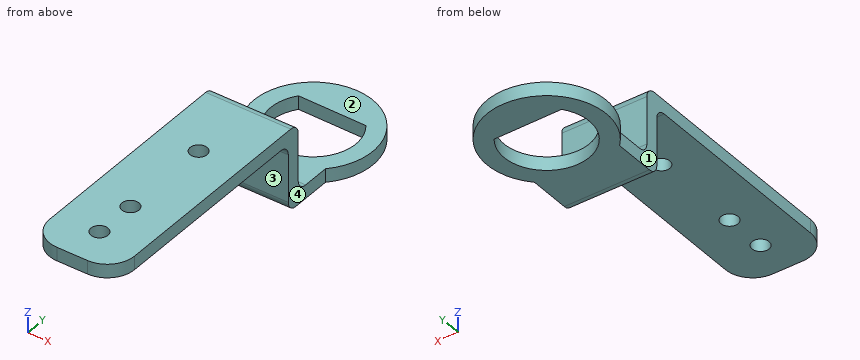
```python
from build123d import *

# Parameters (mm, degrees)
BOSS_EXTRUDE1_DEPTH = 0.4
SKETCH2_W           = 2.5
SKETCH2_H           = 0.4
BOSS_EXTRUDE2_DEPTH = 2
SKETCH3_W           = 2.5
SKETCH3_H           = 0.4
BOSS_EXTRUDE3_DEPTH = 7
FILLET1_R           = 0.3
FILLET2_R           = 0.8
SKETCH4_R           = 0.25
CUT_EXTRUDE1_DEPTH  = 4


with BuildPart() as part:
    # Sketch1 → Boss-Extrude1 (new body)
    with BuildSketch(Plane.XY):
        with BuildLine():
            Line((0.266025337, -2.019252852), (0.266025337, -3.519252852))
            Line((0.266025337, -3.519252852), (2.766025337, -3.519252852))
            Line((2.766025337, -3.519252852), (2.766025337, -2.019252852))
            ThreePointArc((2.766025337, -2.019252852), (1.516025337, 0.955492019), (0.266025337, -2.019252852))
        make_face()
        with BuildLine():
            Line((2.524676695, -0.056183906), (0.524811845, -0.032933419))
            ThreePointArc((0.524811845, -0.032933419), (1.501493783, -2.044423511), (2.524676695, -0.056183906))
        make_face(mode=Mode.SUBTRACT)
    extrude(amount=BOSS_EXTRUDE1_DEPTH)

    # Sketch2 → Boss-Extrude2 (add)
    with BuildSketch(Plane.XY.offset(0.4)):
        with Locations((1.516025337, -3.319252852)):
            Rectangle(SKETCH2_W, SKETCH2_H)
    extrude(amount=BOSS_EXTRUDE2_DEPTH)

    # Sketch3 → Boss-Extrude3 (add)
    with BuildSketch(Plane.XZ.offset(3.519252852)):
        with Locations((1.516025337, 2.2)):
            Rectangle(SKETCH3_W, SKETCH3_H)
    extrude(amount=BOSS_EXTRUDE3_DEPTH)

    # Fillet1
    fillet1_edges = [part.edges().sort_by_distance(p)[0] for p in [
        (1.516025337, -3.119252852, 0.4),
        (1.516025337, -3.119252852, 2.4),
        (1.516025337, -3.519252852, 2),
        (1.516025337, -3.519252852, 0),
    ]]
    fillet(fillet1_edges, radius=FILLET1_R)

    # Fillet2
    fillet2_edges = [part.edges().sort_by_distance(p)[0] for p in [
        (0.266025337, -10.519252852, 2.2),
        (2.766025337, -10.519252852, 2.2),
    ]]
    fillet(fillet2_edges, radius=FILLET2_R)

    # Sketch4 → Cut-Extrude1 (cut)
    with BuildSketch(Plane.XY.offset(2.4)):
        with Locations((1.516025337, -5.419252852)):
            Circle(SKETCH4_R)
        with Locations((1.516025337, -9.419252852)):
            Circle(SKETCH4_R)
        with Locations((1.516025337, -8.169252852)):
            Circle(SKETCH4_R)
    extrude(amount=-CUT_EXTRUDE1_DEPTH, mode=Mode.SUBTRACT)


solid = part.part
```
Check sheet for the modelled part. Datum: model origin and axes. Units: mm. Face numbers are marked on the shaded views. A direction names the side the tool comes from. Coordinates: 2 decimals unless noted, no trailing zeros. Order: outer loops, then holes, each group sorted by start corner. A loop starts at its lowest first (then second) coordinate and runs counter-clockwise, first axis right, second up. Notation, with made-up numbers: M 82.25,57 L 111.25,57 A22 cw 111.25,83 Z; hole C -35,-31.5 d10. An arc over 180 degrees is marked long. Write each question's results on one line, items separated by ' | '. Start each with the question number.
1. Cross-section at C-C on x = 0.4. Record the cut outline in (y, z), and give its area (3 significant figures).
2. Go/stop test with flat-tipped pins: P1, Ø1, axis at x = 2.5, z = 0.5, coming from the -Y side; P2, Ø1, axis at x = 1.5, y = -1.5, coming from the +Z side. Record where each tip stops, or that it passes through.
3. Cross-section at A-A on x = 1.55. Record the cut outline in (y, z), and give its area (3 significant figures).
4. Cross-section at B-B on y = -1. Record the cut outline in (x, z).
5. Cross-section at D-D on y = -6. Record the cut outline in (x, z), and give its area (3 significant figures).
6. Access from +Z, -Z, +X, -X, +Y, -Y to the whole of each face (thin tool, end or side, straight path). Record for the marked faces 1, 2, 3 and 4.
7. Material ranges on probe 1 along Y at (x, z) = (0.5, 1); probe 2 along Z at (x, y) = (0.4, -2.5); probe 3 along Z at (x, y) = (2.5, -8), recorded low to high.
Checks:
1) outline: M -10.16,2 L -3.82,2 A0.3 cw -3.52,1.7 L -3.52,0.3 A0.3 ccw -3.22,0 L -1.36,0 L -1.36,0.4 L -2.82,0.4 A0.3 cw -3.12,0.7 L -3.12,2.1 A0.3 ccw -3.42,2.4 L -10.16,2.4 Z; M -0.23,0 L 0.55,0 L 0.55,0.4 L -0.23,0.4 Z | area: 4.64 mm²
2) P1: stops at y = -3.52 | P2: passes through
3) outline: M -10.52,2 L -9.67,2 L -9.67,2.4 L -10.52,2.4 Z; M -9.17,2 L -8.42,2 L -8.42,2.4 L -9.17,2.4 Z; M -7.92,2 L -5.67,2 L -5.67,2.4 L -7.92,2.4 Z; M -5.17,2 L -3.82,2 A0.3 cw -3.52,1.7 L -3.52,0.3 A0.3 ccw -3.22,0 L -2.04,0 L -2.04,0.4 L -2.82,0.4 A0.3 cw -3.12,0.7 L -3.12,2.1 A0.3 ccw -3.42,2.4 L -5.17,2.4 Z; M -0.04,0 L 0.96,0 L 0.96,0.4 L -0.04,0.4 Z | area: 4.00 mm²
4) outline: M -0.22,0 L 0.28,0 L 0.28,0.4 L -0.22,0.4 Z; M 2.75,0 L 3.25,0 L 3.25,0.4 L 2.75,0.4 Z
5) outline: M 0.27,2 L 2.77,2 L 2.77,2.4 L 0.27,2.4 Z | area: 1.00 mm²
6) face 1: +Z, -Z, -X, -Y | face 2: +Z, +X, -X, +Y | face 3: -Z, +X, -X, -Y | face 4: +Z, -Z, +X, -Y
7) probe 1: y = -3.52 to -3.12 | probe 2: z = 0 to 0.4 | probe 3: z = 2 to 2.4
